```python
from build123d import *

# Parameters (mm, degrees)
BOSS_EXTRUDE1_DEPTH = 3
SKETCH2_R           = 4
CUT_EXTRUDE1_DEPTH  = 13
BOSS_EXTRUDE2_DEPTH = 15.5
SKETCH6_R           = 4.6
CUT_EXTRUDE4_DEPTH  = 1.5
SKETCH7_R           = 2
CUT_EXTRUDE5_DEPTH  = 10
SKETCH8_R           = 1
CUT_EXTRUDE6_DEPTH  = 10
SKETCH4_R           = 1
CUT_EXTRUDE9_DEPTH  = 3
SKETCH11_R          = 1
CUT_EXTRUDE11_DEPTH = 3
SKETCH12_W          = 2.5
SKETCH12_H          = 7
BOSS_EXTRUDE3_DEPTH = 6
SKETCH13_R          = 1
CUT_EXTRUDE12_DEPTH = 6
FILLET1_R           = 2


with BuildPart() as part:
    # Sketch1 → Boss-Extrude1 (new body)
    with BuildSketch(Plane(origin=(0, 0, 0), x_dir=(1, 0, 0), z_dir=(0, 1, 0))):
        with BuildLine():
            Line((-10, 0), (-14, -20))
            Line((-14, -20), (14, -20))
            Line((14, -20), (10, 0))
            ThreePointArc((10, 0), (0, 10), (-10, 0))
        make_face()
    extrude(amount=BOSS_EXTRUDE1_DEPTH)

    # Sketch2 → Cut-Extrude1 (cut)
    with BuildSketch(Plane(origin=(0, 3, 0), x_dir=(1, 0, 0), z_dir=(0, 1, 0))):
        Circle(SKETCH2_R)
    extrude(amount=-CUT_EXTRUDE1_DEPTH, mode=Mode.SUBTRACT)

    # Sketch5 → Boss-Extrude2 (add)
    with BuildSketch(Plane(origin=(0, 3, 0), x_dir=(1, 0, 0), z_dir=(0, 1, 0))):
        Polygon((-13.4, -17), (13.4, -17), (14, -20), (-14, -20), align=None)
    extrude(amount=BOSS_EXTRUDE2_DEPTH)

    # Sketch6 → Cut-Extrude4 (cut)
    with BuildSketch(Plane(origin=(0, 3, 0), x_dir=(1, 0, 0), z_dir=(0, 1, 0))):
        Circle(SKETCH6_R)
    extrude(amount=-CUT_EXTRUDE4_DEPTH, mode=Mode.SUBTRACT)

    # Sketch7 → Cut-Extrude5 (cut)
    with BuildSketch(Plane(origin=(0, 3, 0), x_dir=(1, 0, 0), z_dir=(0, 1, 0))):
        with Locations((-7.071067812, 7.071067812)):
            Circle(SKETCH7_R)
        with Locations((7.071067812, 7.071067812)):
            Circle(SKETCH7_R)
    extrude(amount=-CUT_EXTRUDE5_DEPTH, mode=Mode.SUBTRACT)

    # Sketch8 → Cut-Extrude6 (cut)
    with BuildSketch(Plane(origin=(0, 0, 17), x_dir=(-1, 0, 0), z_dir=(0, 0, -1))):
        with Locations((-6.69393863, 7.151837118)):
            Circle(SKETCH8_R)
        with Locations((-6.69393863, 14.651837118)):
            Circle(SKETCH8_R)
        with Locations((7.30606137, 14.651837118)):
            Circle(SKETCH8_R)
        with Locations((7.073668949, 7.151837118)):
            Circle(SKETCH8_R)
    extrude(amount=-CUT_EXTRUDE6_DEPTH, mode=Mode.SUBTRACT)

    # Sketch4 → Cut-Extrude9 (cut)
    with BuildSketch(Plane(origin=(0, 3, 0), x_dir=(1, 0, 0), z_dir=(0, 1, 0))):
        with Locations((-7, 0)):
            Circle(SKETCH4_R)
    extrude(amount=-CUT_EXTRUDE9_DEPTH, mode=Mode.SUBTRACT)

    # Sketch11 → Cut-Extrude11 (cut)
    with BuildSketch(Plane(origin=(0, 3, 0), x_dir=(1, 0, 0), z_dir=(0, 1, 0))):
        with Locations((0, -7.597940957)):
            Circle(SKETCH11_R)
        with Locations((7.256224789, 0)):
            Circle(SKETCH11_R)
    extrude(amount=-CUT_EXTRUDE11_DEPTH, mode=Mode.SUBTRACT)

    # Sketch12 → Boss-Extrude3 (add)
    with BuildSketch(Plane.XZ):
        with Locations((0, 14.439281905)):
            Rectangle(SKETCH12_W, SKETCH12_H)
    extrude(amount=BOSS_EXTRUDE3_DEPTH)

    # Sketch13 → Cut-Extrude12 (cut)
    with BuildSketch(Plane.ZY.offset(1.25)):
        with Locations((14.409447897, -3)):
            Circle(SKETCH13_R)
    extrude(amount=-CUT_EXTRUDE12_DEPTH, mode=Mode.SUBTRACT)

    # Fillet1
    fillet1_edges = [part.edges().sort_by_distance(p)[0] for p in [
        (0, -6, 17.939281905),
        (0, 0, 10.939281905),
        (0, 0, 17.939281905),
        (0, -6, 10.939281905),
    ]]
    fillet(fillet1_edges, radius=FILLET1_R)


solid = part.part
```
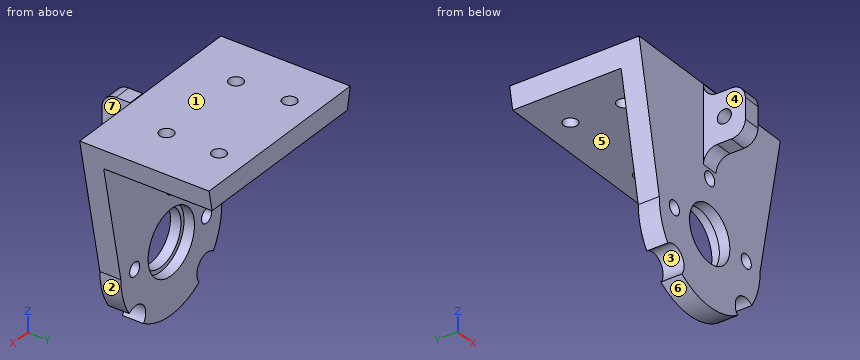
For this review, take the finished solid that the model builds, in its own axes (mm). Face numbers are marked on the shaded views. A direction names the side the tool comes from. Coordinates: 2 decimals unless noted, no trailing zeros. Loops run counter-clockwise (first coordinate to the right, second up) from the corner with the lowest first, then second, coordinate; pieces in that order, holes last.
1. Insertion check: P1, Ø2.5, axis at x = 6.69, y = 14.65, coming from the -Z side; P2, Ø1.8, axis at x = 6.69, y = 7.15, coming from the +Z side; P3, Ø10.5, axis at x = 0, z = 0, coming from the +Y side; P4, Ø3, axis at x = 7, z = 1, coming from the -Y side. Each pin has a flat end and moves straight along its axis. Give the tip position at first contact, or say it passes through.
2. For the marked faces 5, 6 and 7, list the 3-axis set-ups (+Z, -Z, +X, -X, +Y, -Y) from which the entire face can be reached by the end or side of a thin tool; tool diameter is ignored.
3. Add section C-C, the plane z = 7. Give the boundary of the cut face in (x, y), then the cut area to 3 significant figures.
4. Add section B-B, the plane y = -3. Give the boundary of the cut face in (x, z), then the cut area to 3 significant figures.
5. Mouldability with a two-part tool opening along Z and no side actions: class the marked faces 1, 2, 3 and 4 as +Z half, -Z half, draft (parallel to the pull), parting line (faces both ways), or undercut.
6. Add section A-A, the plane x = 0. Give the boundary of the cut face in (y, z).
7. For line 1 (X direction, y = 0.9, z = 0); line 2 (X direction, y = 2, z = 0); line 3 (Y direction, x = 6.75, z = 18.5), list the stretches that pass through material, from the lowest coordinate up.
8. Add section D-D, the plane x = 3.5. Give the boundary of the cut face in (y, z).
Result:
1. P1: stops at z = 17
1. P2: passes through
1. P3: stops at y = 3
1. P4: stops at y = 0
2. face 5: -Z, +X, -X, +Y
2. face 6: -Z, +Y, -Y
2. face 7: +Z, -Z, +X, -Y
3. outline: (-11.4, 0) - (-0.8, 0) - (-0.8, 3) - (-11.4, 3) - close; (0.8, 0) - (11.4, 0) - (11.4, 3) - (0.8, 3) - close
3. area: 63.6 mm2
4. outline: (-1.25, 10.94) - (1.25, 10.94) - (1.25, 13.41) - (-1.25, 13.41) - close; (-1.25, 15.41) - (1.25, 15.41) - (1.25, 17.94) - (-1.25, 17.94) - close
4. area: 12.5 mm2
5. face 1: +Z half
5. face 2: -Z half
5. face 3: undercut
5. face 4: draft
6. outline: (-6, 12.94) arc R2 ccw to (-4, 10.94) - (-2, 10.94) arc R2 cw to (0, 8.94) - (0, 8.6) - (3, 8.6) - (3, 17) - (18.5, 17) - (18.5, 20) - (0, 20) - (0, 19.94) arc R2 cw to (-2, 17.94) - (-4, 17.94) arc R2 ccw to (-6, 15.94) - close; (0, -10) - (3, -10) - (3, -4.6) - (1.5, -4.6) - (1.5, -4) - (0, -4) - close; (0, 4) - (1.5, 4) - (1.5, 4.6) - (3, 4.6) - (3, 6.6) - (0, 6.6) - close; hole circle Ø2 at (-3, 14.41)
7. line 1: x = -10 to -8, -6 to -4, 4 to 6.26, 8.26 to 10
7. line 2: x = -10 to -8, -6 to -4.6, 4.6 to 6.26, 8.26 to 10
7. line 3: y = 0 to 6.15, 8.15 to 13.65, 15.65 to 18.5
8. outline: (0, -9.37) - (3, -9.37) - (3, -2.98) - (1.5, -2.98) - (1.5, -1.94) - (0, -1.94) - close; (0, 1.94) - (1.5, 1.94) - (1.5, 2.98) - (3, 2.98) - (3, 17) - (18.5, 17) - (18.5, 20) - (0, 20) - close
